from build123d import *

# Parameters (mm, degrees)
SKETCH_1_W                         = 90
SKETCH_1_H                         = 70.2
SM_BASE_FLANGE_1_DEPTH             = 2
SM_EDGE_FLANGE_1_STRIP_W           = 9.4732
SM_EDGE_FLANGE_1_STRIP_H           = 2
SM_EDGE_FLANGE_1_STRIP_CUT_DEPTH   = 90
SM_EDGE_FLANGE_1_STRIP_2_W         = 9.4732
SM_EDGE_FLANGE_1_STRIP_2_H         = 2
SM_EDGE_FLANGE_1_STRIP_CUT_2_DEPTH = 90
SM_EDGE_FLANGE_1_DEPTH             = 90
SM_EDGE_FLANGE_1_BEND_DEPTH        = 90
SKETCH_12_W                        = 50.800050643
SKETCH_12_H                        = 4.268431417
CUT_EXTRUDE_1_DEPTH                = 10
FILLET_1_R                         = 1
FILLET_2_R                         = 1
HOLE_WIZARD_M2_5_2_D               = 2.9
HOLE_WIZARD_M3_1_D                 = 3.4


# Sheet-metal steps are written as plain solids
with BuildPart() as part:
    # Sketch 1 → 基体-法兰1 (new body)
    with BuildSketch(Plane(origin=(0, 0, 0), x_dir=(1, 0, 0), z_dir=(0, 1, 0))):
        Rectangle(SKETCH_1_W, SKETCH_1_H)
    extrude(amount=-SM_BASE_FLANGE_1_DEPTH)

    # 边线-法兰1 strip (across the edge) → 边线-法兰1 strip cut (cut)
    with BuildSketch(Plane(origin=(-45, 0, 35.1), x_dir=(0, 0, -1), z_dir=(1, 0, 0))):
        with Locations((-2, -1)):
            Rectangle(SM_EDGE_FLANGE_1_STRIP_W, SM_EDGE_FLANGE_1_STRIP_H)
    extrude(amount=SM_EDGE_FLANGE_1_STRIP_CUT_DEPTH, mode=Mode.SUBTRACT)

    # 边线-法兰1 strip 2 (across the edge) → 边线-法兰1 strip cut 2 (cut)
    with BuildSketch(Plane(origin=(45, 0, -35.1), x_dir=(0, 0, 1), z_dir=(-1, 0, 0))):
        with Locations((-2, -1)):
            Rectangle(SM_EDGE_FLANGE_1_STRIP_2_W, SM_EDGE_FLANGE_1_STRIP_2_H)
    extrude(amount=SM_EDGE_FLANGE_1_STRIP_CUT_2_DEPTH, mode=Mode.SUBTRACT)

    # 边线-法兰1 section (across the edge) → 边线-法兰1 (add)
    with BuildSketch(Plane(origin=(-45, 0, 35.1), x_dir=(0, 0, -1), z_dir=(1, 0, 0))):
        with BuildLine():
            Line((0, 0.7366), (0, 8))
            Line((0, 8), (2, 8))
            Line((2, 8), (2, 0.7366))
            ThreePointArc((2, 0.7366), (2.215745145, 0.215745145), (2.7366, 0))
            Line((2.7366, 0), (2.7366, -2))
            ThreePointArc((2.7366, -2), (0.801531583, -1.198468417), (0, 0.7366))
        make_face()
    extrude(amount=SM_EDGE_FLANGE_1_DEPTH)

    # 边线-法兰1 section 2 (across the edge) → 边线-法兰1 bend (add)
    with BuildSketch(Plane(origin=(45, 0, -35.1), x_dir=(0, 0, 1), z_dir=(-1, 0, 0))):
        with BuildLine():
            Line((0, 0.7366), (0, 8))
            Line((0, 8), (2, 8))
            Line((2, 8), (2, 0.7366))
            ThreePointArc((2, 0.7366), (2.215745145, 0.215745145), (2.7366, 0))
            Line((2.7366, 0), (2.7366, -2))
            ThreePointArc((2.7366, -2), (0.801531583, -1.198468417), (0, 0.7366))
        make_face()
    extrude(amount=SM_EDGE_FLANGE_1_BEND_DEPTH)

    # 草图12 → 切除-拉伸1 (cut)
    with BuildSketch(Plane(origin=(0, 0, 0), x_dir=(1, 0, 0), z_dir=(0, 1, 0))):
        with Locations((-8.635838808, 29.089367058)):
            Rectangle(SKETCH_12_W, SKETCH_12_H)
    extrude(amount=-CUT_EXTRUDE_1_DEPTH, mode=Mode.SUBTRACT)

    # 圆角1
    fillet_1_edges = [part.edges().sort_by_distance(p)[0] for p in [
        (-34.035864129, -1, -26.955151349),
        (-34.035864129, -1, -31.223582766),
        (16.764186514, -1, -31.223582766),
        (16.764186514, -1, -26.955151349),
    ]]
    fillet(fillet_1_edges, radius=FILLET_1_R)

    # 圆角2
    fillet_2_edges = [part.edges().sort_by_distance(p)[0] for p in [
        (-45, 8, 34.1),
        (45, 8, 34.1),
        (45, 8, -34.1),
        (-45, 8, -34.1),
    ]]
    fillet(fillet_2_edges, radius=FILLET_2_R)

    # M2.5 间隙孔2 (through all)
    with Locations(Plane.XY.offset(35.1)):
        with Locations((0, 4.5), (35, 4.5), (-35, 4.5)):
            Hole(HOLE_WIZARD_M2_5_2_D / 2)

    # M3 间隙孔1 (through all)
    with Locations(Plane(origin=(0, 0, 0), x_dir=(1, 0, 0), z_dir=(0, 1, 0))):
        with Locations((-37.464896876, -24.56505715), (-37.464896876, 24.542151638), (20.447218948, 24.542151638), (20.447218948, -24.479946406)):
            Hole(HOLE_WIZARD_M3_1_D / 2)


solid = part.part
Here's how the part is built. I have some questions about the finished solid (model axes, mm). A direction names the side the tool comes from. Coordinates: 2 decimals unless noted, no trailing zeros. Write each loop counter-clockwise with the first axis right and the second up, starting at its lowest first coordinate (ties: lowest second). Pieces come first, ordered by that corner, then holes.
1) If we section it at C-C (z = -29): List the corners of the cut face in (x, y) for me, plus the area to 3 significant figures.
Filled in:
outline: (-45, -2) - (-34.04, -2) - (-34.04, 0) - (-45, 0) - close; (16.76, -2) - (45, -2) - (45, 0) - (16.76, 0) - close
area: 78.4 mm2
2) If we section it at B-B (y = 4.5): Count the separate pieces of the cut face and the enclosed holes in it, plus the area to 3 significant figures.
Filled in:
separate pieces: 8
enclosed holes: 0
area: 325 mm2
3) Which directions (+Z, -Z, +X, -X, +Y, -Y) give clear straight access to the entire face, cutting with the end or side of a thin tool? Please do faces 5 (the face through (-45, -1, 0)), 6 (the face through (16.764, -1, -29)), 7 (the face through (-1, 0, 0)).
Filled in:
face 5: +Z, -Z, -X, +Y, -Y
face 6: +Y, -Y
face 7: +X, -X, +Y
4) I'm going to push flat-ended pins straight in: pin 1 (1.6 mm diameter, centred on x = -18.5, y = -1, fed in from -Z); pin 2 (5.5 mm diameter, centred on x = -37.46, z = 24.57, fed in from +Y); pin 3 (1 mm diameter, centred on x = -6, y = -1.5, fed in from +Z). Where does each tip first touch, or does it pass through?
Filled in:
pin 1: stops at z = -34.93
pin 2: stops at y = 0
pin 3: stops at z = 34.48
5) If we section it at A-A (x = -26): List the corners of the cut face in (y, z) for me.
Filled in:
outline: (-2, -32.36) arc R2.74 ccw to (0.74, -35.1) - (8, -35.1) - (8, -33.1) - (0.74, -33.1) arc R0.74 cw to (0, -32.36) - (0, -31.22) - (-2, -31.22) - close; (-2, -26.96) - (0, -26.96) - (0, 32.36) arc R0.74 cw to (0.74, 33.1) - (8, 33.1) - (8, 35.1) - (0.74, 35.1) arc R2.74 ccw to (-2, 32.36) - close
6) If we section it at D-D (x = 0): List the corners of the cut face in (y, z) for me, plus the area to 3 significant figures.
Filled in:
outline: (-2, -32.36) arc R2.74 ccw to (0.74, -35.1) - (3.05, -35.1) - (3.05, -33.1) - (0.74, -33.1) arc R0.74 cw to (0, -32.36) - (0, -31.22) - (-2, -31.22) - close; (-2, -26.96) - (0, -26.96) - (0, 32.36) arc R0.74 cw to (0.74, 33.1) - (3.05, 33.1) - (3.05, 35.1) - (0.74, 35.1) arc R2.74 ccw to (-2, 32.36) - close; (5.95, -35.1) - (8, -35.1) - (8, -33.1) - (5.95, -33.1) - close; (5.95, 33.1) - (8, 33.1) - (8, 35.1) - (5.95, 35.1) - close
area: 149 mm2
7) Thinking about a two-plate mould opening in X: for faces 1 (the face through (-1, 3, 33.1)), 2 (the face through (-33.55, 4.56, 34.09)), 3 (the face through (-9, -1, -31.224)), 4 (the face through (45, -1, 0)), which applies, +X half, -X half, draft (parallel to the pull), parting line (faces both ways), or undercut?
Filled in:
face 1: draft
face 2: undercut
face 3: undercut
face 4: +X half
8) If I drill on line 1 (Z direction, x = 37.5, y = 4.75); line 2 (Y direction, x = 26, z = 32); line 3 (Z direction, x = -25.5, y = -0.5), over which ranges is the centre line in solid material (lowest first)?
Filled in:
line 1: z = -35.1 to -33.1, 33.1 to 35.1
line 2: y = -2 to 0
line 3: z = -34.8 to -31.22, -26.96 to 34.8
